Verification items for the finished model (mm, model axes). A direction names the side the tool comes from. Coordinates: 2 decimals unless noted, no trailing zeros. Order: outer loops, then holes, each group sorted by start corner. A loop starts at its lowest first (then second) coordinate and runs counter-clockwise, first axis right, second up. Notation, with made-up numbers: (-22, 69.25) -> (31, 69.25) arc R25 cw to (31, 95.25) -> close; hole circle Ø11 at (63, 43.5). An arc over 180 degrees is marked (long way). Use CSV: the item, a comma, the result in double quotes. Start each with the question number.
1) Go/stop test with flat-tipped pins: pin 1 (11.5 mm diameter, centred on x = 9, y = 16, fed in from +Z); pin 2 (1.5 mm diameter, centred on x = 13, z = 30.5, fed in from +Y). Record where each tip stops, or that it passes through.
2) Sectioned sample at C-C on y = -8. Record the boundary of the cut face in (x, z).
3) Tool access check on faces 4 (the flat face through (74, 37.5, 99)), 5 (the flat face through (-1, 11, 102)), 6 (the flat face through (-1, 12, 15)). Record the directions out of +Z, -Z, +X, -X, +Y, -Y that give a thin tool (end or side, any length) a straight path to the whole face; none if there is none.
4) Release check for a two-part mould opening along X. For faces 1 (the cylindrical face through (-0.615, 14.754, 57.891)), 2 (the flat face through (-1, -37.5, 99)), 3 (the flat face through (100, -1, 99)) record: released by +X, released by -X, zero draft, split by the parting line, or undercut.
5) Scan lines: line 1 along Z through (x, y) = (32, 30); line 2 along X through (y, z) = (12.5, 174); line 3 along X through (y, z) = (22.5, 92). Record each from-to range of solid material in increasing order.
6) Sectioned sample at A-A on y = 28.5. Record the boundary of the cut face in (x, z).
7) Sectioned sample at D-D on z = 128.5. Record the boundary of the cut face in (x, y), then the cut area to 3 significant figures.
8) Sectioned sample at B-B on x = -26.5. Record the boundary of the cut face in (y, z), then the cut area to 3 significant figures.
from build123d import *

# Parameters (mm, degrees)
SKETCH1_W           = 200
SKETCH1_H           = 75
BOSS_EXTRUDE1_DEPTH = 200
CUT_EXTRUDE1_START  = -98
SKETCH2_R           = 52.5
CUT_EXTRUDE1_DEPTH  = 98
CUT_EXTRUDE2_START  = -87
SKETCH3_R           = 37.75
CUT_EXTRUDE2_DEPTH  = 87
SKETCH4_R           = 66
CUT_EXTRUDE3_DEPTH  = 200


with BuildPart() as part:
    # Sketch1 → Boss-Extrude1 (new body)
    with BuildSketch(Plane.XY):
        Rectangle(SKETCH1_W, SKETCH1_H)
    extrude(amount=BOSS_EXTRUDE1_DEPTH)

    # Sketch2 → Cut-Extrude1 (cut)
    with BuildSketch(Plane.XY.offset(200).offset(CUT_EXTRUDE1_START)):
        with Locations((-0.000678119, 52.499321881)):
            Circle(SKETCH2_R)
    extrude(amount=CUT_EXTRUDE1_DEPTH, mode=Mode.SUBTRACT)

    # Sketch3 → Cut-Extrude2 (cut)
    with BuildSketch(Plane.XY.offset(102).offset(CUT_EXTRUDE2_START)):
        with Locations((-0.000678119, 52.499321881)):
            Circle(SKETCH3_R)
    extrude(amount=CUT_EXTRUDE2_DEPTH, mode=Mode.SUBTRACT)

    # Sketch4 → Cut-Extrude3 (cut)
    with BuildSketch(Plane.XY.offset(15)):
        with Locations((-0.000678119, 52.499321881)):
            Circle(SKETCH4_R)
    extrude(amount=-CUT_EXTRUDE3_DEPTH, mode=Mode.SUBTRACT)


solid = part.part
Answers follow:
1,pin 1,"stops at z = 102"
1,pin 2,"stops at y = 17.34"
2,outline,"(-100, 0) -> (-26.38, 0) -> (-26.38, 15) -> (26.38, 15) -> (26.38, 0) -> (100, 0) -> (100, 200) -> (-100, 200) -> close"
3,face 4,"+Z, -Z, +X, -X, +Y"
3,face 5,"+Z, +Y"
3,face 6,"-Z, +Y"
4,face 1,"undercut"
4,face 2,"zero draft"
4,face 3,"released by +X"
5,line 1,"z = 15 to 102"
5,line 2,"x = -100 to -34.01, 34 to 100"
5,line 3,"x = -100 to -22.92, 22.91 to 100"
6,outline,"(-100, 0) -> (-61.48, 0) -> (-61.48, 15) -> (-29.14, 15) -> (-29.14, 102) -> (-46.69, 102) -> (-46.69, 200) -> (-100, 200) -> close; (29.14, 15) -> (61.48, 15) -> (61.48, 0) -> (100, 0) -> (100, 200) -> (46.69, 200) -> (46.69, 102) -> (29.14, 102) -> close"
7,outline,"(-100, -37.5) -> (100, -37.5) -> (100, 37.5) -> (50.31, 37.5) arc R52.5 cw to (-50.31, 37.5) -> (-100, 37.5) -> close"
7,area,"12,200 mm²"
8,outline,"(-37.5, 0) -> (-7.95, 0) -> (-7.95, 15) -> (25.61, 15) -> (25.61, 102) -> (7.18, 102) -> (7.18, 200) -> (-37.5, 200) -> close"
8,area,"10,300 mm²"
